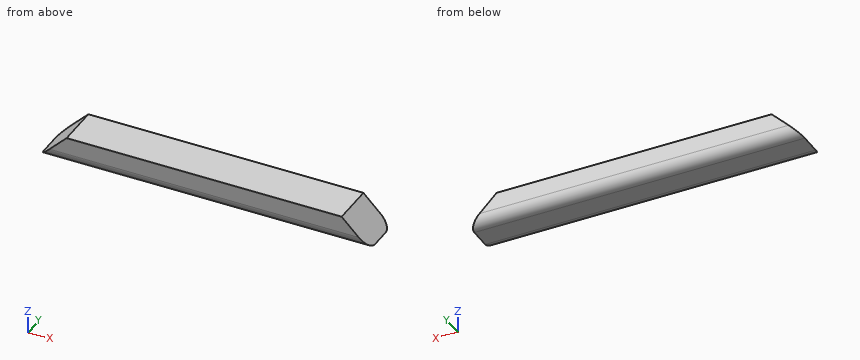
```python
from build123d import *

# Parameters (mm, degrees)
BOSS_EXTRUDE1_DEPTH = 984.25
SKETCH2_W           = 344.402501539
SKETCH2_H           = 493.213131915
CUT_EXTRUDE1_DEPTH  = 59.371664787


with BuildPart() as part:
    # Sketch1 → Boss-Extrude1 (new body)
    with BuildSketch(Plane(origin=(0, 0, 0), x_dir=(0, 0, -1), z_dir=(1, 0, 0))):
        with BuildLine():
            Line((0, 0), (31.75, 0))
            ThreePointArc((31.75, 0), (54.200640303, 9.299359697), (63.5, 31.75))
            Line((63.5, 31.75), (63.5, 95.25))
            ThreePointArc((63.5, 95.25), (54.200640303, 117.700640303), (31.75, 127))
            Line((31.75, 127), (0, 127))
            Line((0, 127), (-19.05, 127))
            Line((-19.05, 127), (-19.05, 0))
            Line((-19.05, 0), (0, 0))
        make_face()
    extrude(amount=BOSS_EXTRUDE1_DEPTH)

    # Sketch2 → Cut-Extrude1 (cut, through all)
    with BuildSketch(Plane(origin=(460.375, 0, 460.375), x_dir=(0, 1, 0), z_dir=(0.707106781, 0, 0.707106781))):
        with Locations((32.995160032, -679.680893327)):
            Rectangle(SKETCH2_W, SKETCH2_H)
    cut_extrude1 = extrude(amount=CUT_EXTRUDE1_DEPTH, mode=Mode.SUBTRACT)

    # Mirror1: Cut-Extrude1 across plane
    add(cut_extrude1.mirror(Plane(origin=(492.125, 0, 0), x_dir=(0, 0, 1), z_dir=(1, 0, 0))), mode=Mode.SUBTRACT)


solid = part.part
```
Work out the finished part from the listing and answer in its coordinate system (mm). Round coordinates to 2 decimals unless told otherwise and drop trailing zeros. Order: outer loops, then holes, each group sorted by start corner. A loop starts at its lowest first (then second) coordinate and runs counter-clockwise, first axis right, second up.
Q1. Given pin 1 Ø10 at (y, z) = (91.5, -14.5) entering from +X; pin 2 Ø8 at (y, z) = (71, -24) entering from +X; pin 3 Ø6 at (x, y) = (205.5, 22) entering from -Z, each flat-ended and moving along its own axis, determine where each tip first touches the part or whether it passes through.
Solution:
pin 1: stops at x = 940.25
pin 2: stops at x = 948.75
pin 3: stops at z = -62.77
Q2. Find the intervals of material crossed by line 1 along Y through (x, z) = (273.5, -34); line 2 along Z through (x, y) = (918, 117.5); line 3 along Y through (x, z) = (754.5, -58), in increasing order.
Solution:
line 1: y = 0.08 to 126.92
line 2: z = -54.4 to 2.75
line 3: y = 13.89 to 113.11
Q3. A cutting plane is placed at B-B, the plane z = 3.5. Determine the outline of the cut face in (x, y), then the cut area to 3 significant figures.
Solution:
outline: (67, 0) - (917.25, 0) - (917.25, 127) - (67, 127) - close
area: 108,000 mm2
Q4. A cutting plane is placed at C-C, the plane y = 51. Determine the outline of the cut face in (x, z).
Solution:
outline: (0, -63.5) - (984.25, -63.5) - (901.7, 19.05) - (82.55, 19.05) - close
Q5. A cutting plane is placed at A-A, the plane x = 846.5. Determine the outline of the cut face in (y, z).
Solution:
outline: (0, -31.75) arc R31.75 ccw to (31.75, -63.5) - (95.25, -63.5) arc R31.75 ccw to (127, -31.75) - (127, 19.05) - (0, 19.05) - close
